from build123d import *

# Parameters (mm, degrees)
SKETCH2_W                   = 100
SKETCH2_H                   = 210
SKETCH2_R                   = 4
BOSS_EXTRUDE1_DEPTH         = 10
SKETCH3_R                   = 2.5
MOUNT_DEPTH                 = 122.346610995
SKETCH7_R                   = 2.5
SUPPORT_PROFILE_MOUNT_DEPTH = 122.346610995
SKETCH4_R                   = 11
SKETCH4_R_2                 = 1.5
STEPPER_MOUNT_DEPTH         = 122.346610995


with BuildPart() as part:
    # Sketch2 → Boss-Extrude1 (new body)
    with BuildSketch(Plane(origin=(0, 0, 0), x_dir=(0, 0, -1), z_dir=(1, 0, 0))):
        with Locations((-10, 0)):
            Rectangle(SKETCH2_W, SKETCH2_H)
        with Locations((0, 88)):
            Circle(SKETCH2_R, mode=Mode.SUBTRACT)
        with Locations(Location((0, 22, 0), (0, 0, 180))):
            Circle(SKETCH2_R, mode=Mode.SUBTRACT)
    extrude(amount=BOSS_EXTRUDE1_DEPTH)

    # Sketch3 → mount (cut, through all)
    with BuildSketch(Plane(origin=(10, 0, 0), x_dir=(0, 0, -1), z_dir=(1, 0, 0))):
        with Locations((-22.5, -70)):
            Circle(SKETCH3_R)
        with Locations(Location((-47.5, -70, 0), (0, 0, 180))):
            Circle(SKETCH3_R)
        with Locations((-47.5, -90)):
            Circle(SKETCH3_R)
        with Locations(Location((-22.5, -90, 0), (0, 0, 180))):
            Circle(SKETCH3_R)
        with Locations((2.5, -90)):
            Circle(SKETCH3_R)
        with Locations(Location((27.5, -90, 0), (0, 0, 180))):
            Circle(SKETCH3_R)
        with Locations((27.5, -70)):
            Circle(SKETCH3_R)
        with Locations(Location((2.5, -70, 0), (0, 0, 180))):
            Circle(SKETCH3_R)
    extrude(amount=-MOUNT_DEPTH, mode=Mode.SUBTRACT)

    # Sketch7 → support_profile_mount (cut, through all)
    with BuildSketch(Plane(origin=(10, 0, 0), x_dir=(0, 0, -1), z_dir=(1, 0, 0))):
        with Locations((-40, 90)):
            Circle(SKETCH7_R)
        with Locations(Location((-40, 20, 0), (0, 0, 180))):
            Circle(SKETCH7_R)
    extrude(amount=-SUPPORT_PROFILE_MOUNT_DEPTH, mode=Mode.SUBTRACT)

    # Sketch4 → stepper_mount (cut, through all)
    with BuildSketch(Plane(origin=(10, 0, 0), x_dir=(0, 0, -1), z_dir=(1, 0, 0))):
        with Locations((0, 55)):
            Circle(SKETCH4_R)
        with Locations((-15.5, 70.5)):
            Circle(SKETCH4_R_2)
        with Locations(Location((15.5, 70.5, 0), (0, 0, 180))):
            Circle(SKETCH4_R_2)
        with Locations(Location((-15.5, 39.5, 0), (0, 0, 180))):
            Circle(SKETCH4_R_2)
        with Locations((15.5, 39.5)):
            Circle(SKETCH4_R_2)
    extrude(amount=-STEPPER_MOUNT_DEPTH, mode=Mode.SUBTRACT)


solid = part.part
Could you check a few things on this model? Use its own coordinates, in mm. Coordinates: 2 decimals unless noted, no trailing zeros. Write each loop counter-clockwise with the first axis right and the second up, starting at its lowest first coordinate (ties: lowest second). Pieces come first, ordered by that corner, then holes. Notation, with made-up numbers: M 4,55 L 48,55 A9 cw 48,60 Z; hole C 89.5,-35.75 d10. An arc over 180 degrees is marked long. One line per question, with ' | ' between items.
1) Imagine slicing it at C-C, the plane z = 8. Write out the boundary of the cut face in (x, y), and give its area (3 significant figures).
Checks:
outline: M 0,-105 L 10,-105 L 10,47.45 L 0,47.45 Z; M 0,62.55 L 10,62.55 L 10,105 L 0,105 Z | area: 1,950 mm²
2) Imagine slicing it at A-A, the plane x = 1.5. Give the number of separate pieces and of enclosed holes in the cut face, and give its area (3 significant figures).
Checks:
separate pieces: 1 | enclosed holes: 17 | area: 20,300 mm²
3) I need wall thicknesses on probe 1 along Y at (x, z) = (7.75, -27.5); probe 2 along Z at (x, y) = (2.75, 70.5); probe 3 along Y at (x, z) = (4.75, 40). Which ranges of each line are inside material? Lowest first, please. Write a range as [from, to].
Checks:
probe 1: [-105, -92.5], [-87.5, -72.5], [-67.5, 105] | probe 2: [-40, -17], [-14, 14], [17, 60] | probe 3: [-105, 17.5], [22.5, 87.5], [92.5, 105]
4) For pin 1 Ø7 at (y, z) = (22, 0) entering from +X, with a flat end and sliding along its axis, tell me the tip position at first contact or that it passes through.
Checks:
pin 1: through
5) Imagine slicing it at D-D, the plane z = 22.5. Write out the boundary of the cut face in (x, y), and give its area (3 significant figures).
Checks:
outline: M 0,-105 L 10,-105 L 10,-92.5 L 0,-92.5 Z; M 0,-87.5 L 10,-87.5 L 10,-72.5 L 0,-72.5 Z; M 0,-67.5 L 10,-67.5 L 10,105 L 0,105 Z | area: 2,000 mm²
6) Imagine slicing it at B-B, the plane y = -90. Write out the boundary of the cut face in (x, z), and give its area (3 significant figures).
Checks:
outline: M 0,-40 L 10,-40 L 10,-30 L 0,-30 Z; M 0,-25 L 10,-25 L 10,-5 L 0,-5 Z; M 0,0 L 10,0 L 10,20 L 0,20 Z; M 0,25 L 10,25 L 10,45 L 0,45 Z; M 0,50 L 10,50 L 10,60 L 0,60 Z | area: 800 mm²
7) If we mould it in two halves opening along Z, with no side actions, what happens to faces 1 (the face through (5, -68, -1)), 2 (the face through (5, -1, -40)), 3 (the face through (10, 1, 11))? For each: released by +Z, released by -Z, zero draft, split by the parting line, or undercut.
Checks:
face 1: undercut | face 2: released by -Z | face 3: zero draft
